Design review of the part built by this model. Coordinates are the model's own, in mm. A direction names the side the tool comes from. Round coordinates to 2 decimals unless told otherwise and drop trailing zeros. Loops run counter-clockwise (first coordinate to the right, second up) from the corner with the lowest first, then second, coordinate; pieces in that order, holes last. Notation, with made-up numbers: (-39, 42.25) -> (-13, 42.25) arc R19 cw to (-13, 50.25) -> close; hole circle Ø1 at (21, 29.25). An arc over 180 degrees is marked (long way). Write each question's results on one line, items separated by ' | '. Start each with the question number.
from build123d import *

# Parameters (mm, degrees)
F0_R     = 6.5
F0_R_2   = 1.75
F3_DEPTH = 20
F4_DEPTH = 30
F5_R     = 3
F6_R     = 5
F7_R     = 16.5
F7_R_2   = 10.70440387
F8_DEPTH = 25


with BuildPart() as f2:
    # F1 (on Right) → F2 (revolve)
    with BuildSketch(Plane.YZ):
        Polygon((12, 20), (12, 0), (35, 0), (35, 20), (30.4406098954, 27.7423450379), align=None)
    revolve(axis=Axis((0, 35.946440883, 0), (0, 1, 0)))

    # F0 (on Front) → F3 (join)
    with BuildSketch(Plane.XZ):
        Circle(F0_R)
        Circle(F0_R_2, mode=Mode.SUBTRACT)
    extrude(amount=-F3_DEPTH)

    # F0 (on Front) → F4 (cut)
    with BuildSketch(Plane.XZ):
        Circle(F0_R_2)
    extrude(amount=-F4_DEPTH, mode=Mode.SUBTRACT)

    # F5
    f5_edges = [f2.edges().sort_by_distance(p)[0] for p in [
        (0, 12, -20),
    ]]
    fillet(f5_edges, radius=F5_R)

    # F6
    f6_edges = [f2.edges().sort_by_distance(p)[0] for p in [
        (0, 30.44061, -27.742345),
    ]]
    fillet(f6_edges, radius=F6_R)

    # F7 (on Front) → F8 (cut)
    with BuildSketch(Plane.XZ):
        Circle(F7_R)
        Circle(F7_R_2, mode=Mode.SUBTRACT)
    extrude(amount=-F8_DEPTH, mode=Mode.SUBTRACT)


solid = f2.part
1) Insertion check: pin 1 (1 mm diameter, centred on x = 11, z = -17.5, fed in from -Y); pin 2 (10 mm diameter, centred on x = 15.5, y = 17.5, fed in from +Z); pin 3 (5 mm diameter, centred on x = -10.5, y = 23, fed in from +Z); pin 4 (4 mm diameter, centred on x = 0, z = 0, fed in from -Y). Each pin has a flat end and moves straight along its axis. Give the tip position at first contact, or say it passes through.
2) The part is to be moulded in two halves that separate along Z. For faces 3 (the face through (-5, 12, 5)), 4 (the face through (1.617, 14.79, -0.67)), 5 (the face through (-7.89, 18.409, 7.235)), 6 (the face through (-5.158, 5.916, -3.955)), say which applies: +Z half, -Z half, draft (parallel to the pull), parting line (faces both ways), or undercut.
3) Take a section at A-A (y = 18). Write out the cut boundary in (x, z), plus the area to 3 significant figures.
4) To check wall thickness, follow line 1 (X direction, y = 22, z = -4); line 2 (Z direction, x = 0, y = 22); line 3 (X direction, y = 13.5, z = 7.5). State the ranges of each line that lie inside material, in increasing order. Write a range as from..to.
5) For faces 1 (the face through (0, 35, 0)), 2 (the face through (11, 25, 0)), list the 3-axis set-ups (+Z, -Z, +X, -X, +Y, -Y) from which the entire face can be reached by the end or side of a thin tool; tool diameter is ignored.
6) Take a section at B-B (y = 5). Write out the cut boundary in (x, z).
Geometry check:
1) pin 1: stops at y = 12.92 | pin 2: stops at z = 20.58 | pin 3: stops at z = 23.82 | pin 4: stops at y = 0
2) face 3: draft | face 4: undercut | face 5: undercut | face 6: parting line
3) outline: circle Ø45.04 at (0, 0); circle Ø21.41 at (0, 0); hole circle Ø33 at (0, 0); hole circle Ø3.5 at (0, 0) | area: 1,090 mm^2
4) line 1: x = -23.87..-16.01, -9.93..9.93, 16.01..23.87 | line 2: z = -24.2..-16.5, -10.7..-1.75, 1.75..10.7, 16.5..24.2 | line 3: x = -19.19..-14.7, -7.64..7.64, 14.7..19.19
5) face 1: +Z, -Z, +X, -X, +Y | face 2: -Y
6) outline: circle Ø13 at (0, 0); hole circle Ø3.5 at (0, 0)
